Check sheet for the modelled part. Datum: model origin and axes. Units: mm. A direction names the side the tool comes from. Give positions to 0.01 mm unless a question says otherwise; leave off trailing zeros. Order: outer loops, then holes, each group sorted by start corner. A loop starts at its lowest first (then second) coordinate and runs counter-clockwise, first axis right, second up.
from build123d import *

# Parameters (mm, degrees)
SKETCH1_R                = 4.5
BOSS_EXTRUDE1_DEPTH      = 2.5
SKETCH2_W                = 10
SKETCH2_H                = 45
BOSS_EXTRUDE2_DEPTH      = 5
CUT_EXTRUDE1_DEPTH       = 147.126229678
CUT_EXTRUDE1_DEPTH_BACK  = 147.126229678
BOSS_EXTRUDE3_DEPTH      = 15.05
FILLET1_R                = 5
FILLET2_R                = 5
BOSS_EXTRUDE4_DEPTH      = 16.5
BOSS_EXTRUDE4_DEPTH_BACK = 2.000004
SKETCH6_W                = 36.1
SKETCH6_H                = 156
SKETCH6_W_2              = 30.1
SKETCH6_H_2              = 150
BOSS_EXTRUDE5_DEPTH      = 5
SKETCH8_W                = 36.1
SKETCH8_H                = 116
BOSS_EXTRUDE6_DEPTH      = 3
CUT_EXTRUDE2_REACH       = 183.097
SKETCH10_W               = 30.1
SKETCH10_H               = 21.5
SKETCH11_W               = 36.1
SKETCH11_H               = 40
CUT_EXTRUDE3_DEPTH       = 5
SKETCH12_W               = 3
SKETCH12_H               = 25
CUT_EXTRUDE4_DEPTH       = 7.5
CUT_EXTRUDE5_REACH       = 195.973
SKETCH13_R               = 3.4
SKETCH14_R               = 6.4
SKETCH14_R_2             = 3.4
BOSS_EXTRUDE7_DEPTH      = 10.5
FILLET3_R                = 3
SKETCH15_W               = 36.1
SKETCH15_H               = 26.5
SKETCH15_W_2             = 30.1
SKETCH15_H_2             = 21.5
BOSS_EXTRUDE8_DEPTH      = 50


with BuildPart() as part:
    # Sketch1 → Boss-Extrude1 (new, symmetric)
    with BuildSketch(Plane(origin=(0, 0, 0), x_dir=(1, 0, 0), z_dir=(0, 1, 0))):
        with BuildLine():
            Line((-31.821067812, 7.071067812), (-7.071067812, 31.821067812))
            ThreePointArc((-7.071067812, 31.821067812), (0, 34.75), (7.071067812, 31.821067812))
            Line((7.071067812, 31.821067812), (31.821067812, 7.071067812))
            ThreePointArc((31.821067812, 7.071067812), (34.75, 0), (31.821067812, -7.071067812))
            Line((31.821067812, -7.071067812), (7.071067812, -31.821067812))
            ThreePointArc((7.071067812, -31.821067812), (0, -34.75), (-7.071067812, -31.821067812))
            Line((-7.071067812, -31.821067812), (-31.821067812, -7.071067812))
            ThreePointArc((-31.821067812, -7.071067812), (-34.75, 0), (-31.821067812, 7.071067812))
        make_face()
        with Locations(Location((0, 24.75, 0), (0, 0, 270))):
            Circle(SKETCH1_R, mode=Mode.SUBTRACT)
        with Locations(Location((24.75, 0, 0), (0, 0, 270))):
            Circle(SKETCH1_R, mode=Mode.SUBTRACT)
        with Locations(Location((0, -24.75, 0), (0, 0, 270))):
            Circle(SKETCH1_R, mode=Mode.SUBTRACT)
        with Locations(Location((-24.75, 0, 0), (0, 0, 270))):
            Circle(SKETCH1_R, mode=Mode.SUBTRACT)
    extrude(amount=BOSS_EXTRUDE1_DEPTH, both=True)


with BuildPart() as body_2:
    # Mirror3: mirrored copy
    add(part.part.mirror(Plane.XY.offset(49.5)))


with BuildPart() as body_3:
    # Sketch2 → Boss-Extrude2 (new, symmetric)
    with BuildSketch(Plane(origin=(0, 0, 0), x_dir=(0, 0, -1), z_dir=(1, 0, 0))):
        with Locations((-99, 25)):
            Rectangle(SKETCH2_W, SKETCH2_H)
    extrude(amount=BOSS_EXTRUDE2_DEPTH, both=True)


with BuildPart() as body_4:
    # Mirror5: mirrored copy
    add(body_3.part.mirror(Plane.XY.offset(49.5)))


with BuildPart() as cut_extrude1_tool:
    # Sketch3 → Cut-Extrude1 (new, two sides: drawn at the far end of the back side and taken through both)
    with BuildSketch(Plane(origin=(0, 0, 0), x_dir=(0, 0, -1), z_dir=(1, 0, 0)).offset(-CUT_EXTRUDE1_DEPTH_BACK)):
        Polygon((-398.060619113, -61.293305417), (-104, 17.5), (5, 46.706461975), (299.060619113, 125.499767392), (141.474008279, 713.621005618), (-555.647229947, 526.827932809), align=None)
    extrude(amount=CUT_EXTRUDE1_DEPTH + CUT_EXTRUDE1_DEPTH_BACK)


with BuildPart() as body_3_1:
    add(body_3.part)

    # Cut-Extrude1: cut by cut_extrude1_tool
    add(cut_extrude1_tool.part, mode=Mode.SUBTRACT)


with BuildPart() as body_4_1:
    add(body_4.part)

    # Cut-Extrude1: cut by cut_extrude1_tool
    add(cut_extrude1_tool.part, mode=Mode.SUBTRACT)

    # Combine2: union part
    add(part.part)

    # Fillet2
    fillet2_edges = [body_4_1.edges().sort_by_distance(p)[0] for p in [
        (-5, 2.5, 0),
        (0, 2.5, 5),
        (0, 2.5, -5),
        (5, 2.5, 0),
    ]]
    fillet(fillet2_edges, radius=FILLET2_R)


with BuildPart() as body_5:
    # Sketch4 → Boss-Extrude3 (new, symmetric)
    with BuildSketch(Plane(origin=(0, 0, 0), x_dir=(0, 0, -1), z_dir=(1, 0, 0))):
        Polygon((-130.821067812, 10.31331654), (14.067806131, 49.136173305), (13.550168041, 51.068024958), (-131.338705902, 12.245168192), align=None)
    extrude(amount=BOSS_EXTRUDE3_DEPTH, both=True)



with BuildPart() as body_2_1:
    add(body_2.part)

    # Combine1: union body 3
    add(body_3_1.part)

    # Fillet1
    fillet1_edges = [body_2_1.edges().sort_by_distance(p)[0] for p in [
        (0, 2.5, 94),
        (5, 2.5, 99),
        (-5, 2.5, 99),
        (0, 2.5, 104),
    ]]
    fillet(fillet1_edges, radius=FILLET1_R)


with BuildPart() as body_5_1:
    add(body_5.part)

    add(body_2_1.part)  # Boss-Extrude4 merges body 2

    add(body_4_1.part)  # Boss-Extrude4 merges body 4
    # Sketch6 → Boss-Extrude4 (add, two sides: drawn at the far end of the back side and taken through both)
    with BuildSketch(Plane(origin=(0, 44.259573936, 11.859317093), x_dir=(1, 0, 0), z_dir=(0, 0.96592582628907, 0.2588190451025143)).offset(-BOSS_EXTRUDE4_DEPTH_BACK)):
        with Locations((0, -48.694165284)):
            Rectangle(SKETCH6_W, SKETCH6_H)
        with Locations((0, -48.694165284)):
            Rectangle(SKETCH6_W_2, SKETCH6_H_2, mode=Mode.SUBTRACT)
    extrude(amount=BOSS_EXTRUDE4_DEPTH + BOSS_EXTRUDE4_DEPTH_BACK)

    # Sketch7 → Boss-Extrude5 (add)
    with BuildSketch(Plane(origin=(0, 60.197350069, 16.129831338), x_dir=(1, 0, 0), z_dir=(0, 0.96592582628907, 0.25881904510251436))):
        Polygon((15.05, 26.305834716), (15.05, -86.694165284), (18.05, -86.694165284), (18.05, 29.305834716), (-18.05, 29.305834716), (-18.05, -86.694165284), (-15.05, -86.694165284), (-15.05, 26.305834716), align=None)
    extrude(amount=BOSS_EXTRUDE5_DEPTH)

    # Sketch8 → Boss-Extrude6 (add)
    with BuildSketch(Plane(origin=(0, 65.026979201, 17.423926563), x_dir=(1, 0, 0), z_dir=(0, 0.96592582628907, 0.25881904510251436))):
        with Locations((0, -28.694165284)):
            Rectangle(SKETCH8_W, SKETCH8_H)
    extrude(amount=BOSS_EXTRUDE6_DEPTH)

    # Sketch10 → Cut-Extrude2 (cut, up to next)
    with BuildSketch(Plane(origin=(0, 6.808451022, -25.409485135), x_dir=(1, 0, 0), z_dir=(0, -0.2588190451025143, 0.96592582628907)), mode=Mode.PRIVATE) as cut_extrude2_sk1:
        with Locations((0, 56.570882651)):
            Rectangle(SKETCH10_W, SKETCH10_H)
    cut_extrude2_tool1 = extrude(cut_extrude2_sk1.sketch, amount=-CUT_EXTRUDE2_REACH, mode=Mode.PRIVATE) & body_5_1.part
    add(cut_extrude2_tool1.solids().sort_by_distance((0, 61.451728, -10.767863))[0], mode=Mode.SUBTRACT)

    # Sketch11 → Cut-Extrude3 (cut)
    with BuildSketch(Plane(origin=(0, 60.197350069, 16.129831338), x_dir=(1, 0, 0), z_dir=(0, 0.96592582628907, 0.25881904510251436))):
        with Locations((0, -106.694165284)):
            Rectangle(SKETCH11_W, SKETCH11_H)
    extrude(amount=-CUT_EXTRUDE3_DEPTH, mode=Mode.SUBTRACT)

    # Sketch12 → Cut-Extrude4 (cut)
    with BuildSketch(Plane(origin=(0, 55.367720938, 14.835736112), x_dir=(1, 0, 0), z_dir=(0, 0.96592582628907, 0.25881904510251447))):
        with Locations((-16.55, -106.694165284)):
            Rectangle(SKETCH12_W, SKETCH12_H)
        with Locations((16.55, -106.694165284)):
            Rectangle(SKETCH12_W, SKETCH12_H)
    extrude(amount=-CUT_EXTRUDE4_DEPTH, mode=Mode.SUBTRACT)

    # Sketch13 → Cut-Extrude5 (cut, up to next)
    with BuildSketch(Plane(origin=(0, -32.790862879, 122.377166288), x_dir=(1, 0, 0), z_dir=(0, -0.2588190451025143, 0.96592582628907)), mode=Mode.PRIVATE) as cut_extrude5_sk1:
        with Locations(Location((0, 50.570882651, 0), (0, 0, 270))):
            Circle(SKETCH13_R)
    cut_extrude5_tool1 = extrude(cut_extrude5_sk1.sketch, amount=-CUT_EXTRUDE5_REACH, mode=Mode.PRIVATE) & body_5_1.part
    add(cut_extrude5_tool1.solids().sort_by_distance((0, 16.056859, 135.465874))[0], mode=Mode.SUBTRACT)

    # Sketch14 → Boss-Extrude7 (add)
    with BuildSketch(Plane(origin=(0, -32.790862879, 122.377166288), x_dir=(1, 0, 0), z_dir=(0, -0.2588190451025143, 0.96592582628907))):
        with Locations(Location((0, 50.570882651, 0), (0, 0, 270))):
            Circle(SKETCH14_R)
        with Locations(Location((0, 50.570882651, 0), (0, 0, 270))):
            Circle(SKETCH14_R_2, mode=Mode.SUBTRACT)
    extrude(amount=BOSS_EXTRUDE7_DEPTH)

    # Fillet3
    fillet3_edges = [body_5_1.edges().sort_by_distance(p)[0] for p in [
        (-16.55, 24.518000898, 129.968458702),
        (-16.55, 30.988477025, 105.820313045),
        (16.55, 24.518000898, 129.968458702),
        (16.55, 30.988477025, 105.820313045),
    ]]
    fillet(fillet3_edges, radius=FILLET3_R)

    # Sketch15 → Boss-Extrude8 (add)
    with BuildSketch(Plane(origin=(0, 7.584908157, -28.307262614), x_dir=(-1, 0, 0), z_dir=(0, 0.2588190451025143, -0.96592582628907))):
        with Locations((0, 57.070882651)):
            Rectangle(SKETCH15_W, SKETCH15_H)
        with Locations((0, 56.570882651)):
            Rectangle(SKETCH15_W_2, SKETCH15_H_2, mode=Mode.SUBTRACT)
    extrude(amount=BOSS_EXTRUDE8_DEPTH)


solid = body_5_1.part
1) Section check A-A, the plane z = 17. State how many separate pieces and enclosed holes the cut face has, then the cut area to 3 significant figures.
Recorded:
separate pieces: 2
enclosed holes: 1
area: 539 mm2
2) Section check D-D, the plane y = 80. Record the cut outline in (x, z), then the cut area to 3 significant figures.
Recorded:
outline: (-18.05, -60.67) - (-15.05, -60.67) - (-15.05, -38.46) - (15.05, -38.46) - (15.05, -60.67) - (18.05, -60.67) - (18.05, -26.87) - (-18.05, -26.87) - close
area: 552 mm2
3) Set-up check for faces 1 (the face through (0.14, 3.37, 7.18)), 2 (the face through (-0.11, 0.04, 133.75)), 3 (the face through (-7.18, 3.37, 98.86)), 4 (the face through (-18.05, 54, 17)): record each of +Z, -Z, +X, -X, +Y, -Y from which the full face is reachable in a straight line by a thin tool's end or side.
Recorded:
face 1: +X, -X
face 2: +Z, -Y
face 3: +Z, -Z, -X
face 4: +Z, -Z, -X, +Y
4) Draft check along Y on faces 5 (the face through (-0.25, 23.04, 135.49)), 6 (the face through (7.18, 3.37, 98.86)), 7 (the face through (-24.552, -0.035, 103.496)). Enter one of: +Y half, -Y half, draft (parallel to the pull), parting line (faces both ways), or undercut.
Recorded:
face 5: +Y half
face 6: undercut
face 7: draft
5) Material ranges on L1, parallel to X at y = -0.95, z = 0; L2, parallel to Z at x = 24, y = 0; L3, parallel to X at y = 62, z = -34, recorded low to high.
Recorded:
L1: x = -34.75 to -29.25, -20.25 to 20.25, 29.25 to 34.75
L2: z = -14.89 to -4.44, 4.44 to 14.89, 84.11 to 94.56, 103.44 to 113.89
L3: x = -18.05 to -15.05, 15.05 to 18.05
6) Section check C-C, the plane x = 24.75. Record the cut outline in (y, z), then the cut area to 3 significant figures.
Recorded:
outline: (-2.5, -14.14) - (2.5, -14.14) - (2.5, -4.5) - (-2.5, -4.5) - close; (-2.5, 4.5) - (2.5, 4.5) - (2.5, 14.14) - (-2.5, 14.14) - close; (-2.5, 84.86) - (2.5, 84.86) - (2.5, 94.5) - (-2.5, 94.5) - close; (-2.5, 103.5) - (2.5, 103.5) - (2.5, 113.14) - (-2.5, 113.14) - close
area: 193 mm2
7) Depth check by flat-ended pin: pin 1 Ø8 at (x, z) = (-15, -36) entering from -Y; pin 2 Ø7 at (x, z) = (24.75, 0) entering from -Y; pin 3 Ø10 at (x, z) = (-10.5, -43) entering from +Y; pin 4 Ø8 at (y, z) = (24.5, 0.5) entering from +X. Enter the tip coordinate at first touch or a pass-through.
Recorded:
pin 1: stops at y = 53.94
pin 2: passes through
pin 3: stops at y = 85.66
pin 4: stops at x = 5
